Input: part model. Units: mm. Frame: model coordinates. Face numbers are marked on the shaded views. Round coordinates to 2 decimals unless told otherwise and drop trailing zeros. Order: outer loops, then holes, each group sorted by start corner. A loop starts at its lowest first (then second) coordinate and runs counter-clockwise, first axis right, second up. Notation, with made-up numbers: (-40, 25.5) -> (-3, 25.5) arc R25 cw to (-3, 52.5) -> close; hole circle Ø4 at (-32, 49.25). An arc over 180 degrees is marked (long way). Use a Markdown table: item, result.
from build123d import *

# Parameters (mm, degrees)
F0_R     = 2.38125
F1_DEPTH = 9.525
F2_R     = 4.8514
F3_DEPTH = 25.4
F4_R     = 1.27
F5_DEPTH = 9.652


with BuildPart() as f1:
    # F0 (on Front) → F1 (new body)
    with BuildSketch(Plane.XZ):
        with BuildLine():
            Line((1.5875, 15.875), (0.7582183389, 7.5821833894))
            ThreePointArc((0.7582183389, 7.5821833894), (5.0844573747, 5.6756227152), (7.4534847176, 1.584287084))
            Line((7.4534847176, 1.584287084), (10.9677938474, 34.7753054223))
            Line((10.9677938474, 34.7753054223), (1.5875, 36.4293043146))
            Line((1.5875, 36.4293043146), (1.5875, 15.875))
        make_face()
        with BuildLine():
            ThreePointArc((0.3159243079, 3.1592430789), (2.354111794, 2.1304418934), (3.175, 0))
            ThreePointArc((3.175, 0), (2.2450640303, -2.2450640303), (0, -3.175))
            ThreePointArc((0, -3.175), (-3.1371548684, -0.4887579481), (-0.965864174, 3.0245216808))
            Line((-0.965864174, 3.0245216808), (-2.3180740176, 7.2588520338))
            ThreePointArc((-2.3180740176, 7.2588520338), (-6.1533780972, 4.4944786119), (-7.62, 0))
            ThreePointArc((-7.62, 0), (0, -7.62), (7.62, 0))
            ThreePointArc((7.62, 0), (7.5782568427, 0.7965068901), (7.4534847176, 1.584287084))
            ThreePointArc((7.4534847176, 1.584287084), (5.0844573747, 5.6756227152), (0.7582183389, 7.5821833894))
            Line((0.7582183389, 7.5821833894), (0.3159243079, 3.1592430789))
        make_face()
        with BuildLine():
            ThreePointArc((-0.3159243079, 3.1592430789), (0, 3.175), (0.3159243079, 3.1592430789))
            Line((0.3159243079, 3.1592430789), (0.7582183389, 7.5821833894))
            ThreePointArc((0.7582183389, 7.5821833894), (0, 7.62), (-0.7582183389, 7.5821833894))
            Line((-0.7582183389, 7.5821833894), (-0.3159243079, 3.1592430789))
        make_face()
        with BuildLine():
            ThreePointArc((-0.965864174, 3.0245216808), (-0.6444244656, 3.1089133324), (-0.3159243079, 3.1592430789))
            Line((-0.3159243079, 3.1592430789), (-0.7582183389, 7.5821833894))
            ThreePointArc((-0.7582183389, 7.5821833894), (-1.5466187175, 7.4613919977), (-2.3180740176, 7.2588520338))
            Line((-2.3180740176, 7.2588520338), (-0.965864174, 3.0245216808))
        make_face()
        with BuildLine():
            ThreePointArc((-7.62, 0), (-6.1533780972, 4.4944786119), (-2.3180740176, 7.2588520338))
            Line((-2.3180740176, 7.2588520338), (-4.9063479519, 15.3638121726))
            ThreePointArc((-4.9063479519, 15.3638121726), (-8.4191710316, 14.2078233352), (-11.6804510943, 12.4641810168))
            Line((-11.6804510943, 12.4641810168), (-7.62, 0))
        make_face()
        with Locations((-6.8576899833, 9.4598067682)):
            Circle(F0_R, mode=Mode.SUBTRACT)
    extrude(amount=F1_DEPTH)

    # F2 (on face) → F3 (join)
    with BuildSketch(Plane(origin=(6.2776469237, 0, 35.6023048685), x_dir=(0.984807753, 0, -0.1736481777), z_dir=(0.1736481777, 0, 0.984807753))):
        with Locations((0, -4.7625)):
            Circle(F2_R)
    extrude(amount=F3_DEPTH)

    # F4
    f4_edges = [f1.edges().sort_by_distance(p)[0] for p in [
        (5.910614, -4.7625, 61.458859),
    ]]
    fillet(f4_edges, radius=F4_R)

    # F0 (on Front) → F5 (cut)
    with BuildSketch(Plane.XZ):
        with Locations((-6.8576899833, 9.4598067682)):
            Circle(F0_R)
    extrude(amount=-F5_DEPTH, mode=Mode.SUBTRACT)


solid = f1.part
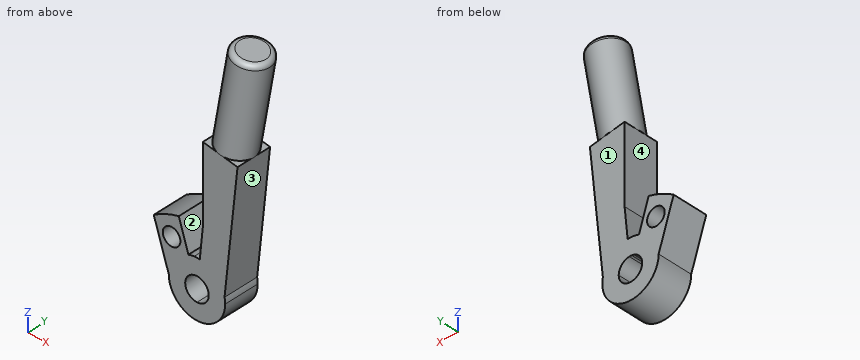
1) Line query: L1, parallel to X at y = -5.5, z = 8; L2, parallel to X at y = -3, z = 9; L3, parallel to Z at x = -1, y = -4. Output: solid intervals per line, ascending. Write a range as [from, to].
Results found:
| item | result |
|---|---|
| L1 | x = [-10.23, -8.74], [-4.98, -2.55], [0.8, 8.13] |
| L2 | x = [-10.55, -9.19], [-4.52, -2.87], [0.9, 8.24] |
| L3 | z = [-7.55, -3.01], [3.01, 7.55] |
2) Cut plane B-B on y = -2.75. Count the separate pieces of the cut face and the enclosed holes in it, and give its area (3 significant figures).
Results found:
| item | result |
|---|---|
| separate pieces | 1 |
| enclosed holes | 2 |
| area | 668 mm² |
3) Pin query (flat end, axial travel): pin 1 Ø7 at (x, z) = (-0.5, 24.5) entering from +Y; pin 2 Ø3 at (x, y) = (-3, -4.5) entering from -Z; pin 3 Ø5 at (x, y) = (4.5, -7) entering from -Z. Return the tip coordinate at first contact, or that it passes through.
Results found:
| item | result |
|---|---|
| pin 1 | stops at y = 0 |
| pin 2 | stops at z = -7.47 |
| pin 3 | stops at z = -7.35 |
4) Pull-direction query (X, two-part tool) for the marked faces 1, 2, 3 and 4; classes: +X half, -X half, draft (parallel to the pull), parting line (faces both ways), or undercut.
Results found:
| item | result |
|---|---|
| face 1 | draft |
| face 2 | undercut |
| face 3 | +X half |
| face 4 | -X half |
5) Cut plane C-C on z = 30.5. Return loops of the section in (x, y) (1 decimal), and give its area (3 significant figures).
Results found:
| item | result |
|---|---|
| outline | (1.6, -9.5) -> (10.5, -9.5) -> (10.5, 0) -> (1.6, 0) -> close |
| area | 85.0 mm² |
6) Cut plane D-D on z = 4. Return loops of the section in (x, y) (3 decimals), and give its area (3 significant figures).
Results found:
| item | result |
|---|---|
| outline | (-8.923, -9.525) -> (7.709, -9.525) -> (7.709, 0) -> (-8.923, 0) -> close |
| area | 158 mm² |
7) Cut plane A-A on x = -6.5. Return loops of the section in (y, z) (3 decimals), and give its area (3 significant figures).
Results found:
| item | result |
|---|---|
| outline | (-9.525, -3.977) -> (0, -3.977) -> (0, 7.106) -> (-9.525, 7.106) -> close; (-9.525, 11.814) -> (0, 11.814) -> (0, 14.923) -> (-9.525, 14.923) -> close |
| area | 135 mm² |
